Work out the finished part from the listing and answer in its coordinate system (mm). A direction names the side the tool comes from. Round coordinates to 2 decimals unless told otherwise and drop trailing zeros. Write each loop counter-clockwise with the first axis right and the second up, starting at its lowest first coordinate (ties: lowest second). Pieces come first, ordered by that corner, then holes.
1. A tool of negligible diameter and unlimited length cuts with its end or side. For faces 4 (the face through (20.35, 1.77, -24.81)), 5 (the face through (-22.72, 4.31, 20.69)), from which of +Z, -Z, +X, -X, +Y, -Y can it reach the whole face along a straight path? Write none if from no direction.
2. Find section D-D (y = 2.8). Write down the section's boundary in (x, z).
3. Find section C-C (x = -21.5). Write down the section's boundary in (y, z), and give its area (3 significant figures).
4. Find section B-B (x = 35). Write down the section's boundary in (y, z), and give its area (3 significant figures).
5. Straight lines are drawn through the part: probe 1 along X at (y, z) = (0.6, -22); probe 2 along X at (y, z) = (1.35, 23); probe 3 along Z at (x, y) = (24, 0.3). For each, find the intervals that lie inside material, in ascending order.
6. Find section A-A (z = -29). Write down the section's boundary in (x, y), and give its area (3 significant figures).
7. Flat-ended cylindrical pins translate along their axes: pin 1 Ø5.5 at (x, z) = (21.5, -22.04) entering from -Y; pin 2 Ø5 at (x, z) = (-35, -29) entering from +Y; pin 3 Ø2 at (x, y) = (-23, 4) entering from -Z. Find the tip coordinate at first contact, or state that the pin passes through.
8. Determine the mould class of faces 1 (the face through (-1, 1, -35)), 2 (the face through (-42.5, 1, 0)), 3 (the face through (34.1, 2.5, -18.7)) for opening direction X: pulls with the +X half, pulls with the -X half, needs draft (parallel to the pull), parting line crosses it, or undercut.
```python
from build123d import *

# Parameters (mm, degrees)
SKETCH1_W           = 85
SKETCH1_H           = 70
SKETCH1_R           = 1.5
BOSS_EXTRUDE1_DEPTH = 5
CUT_EXTRUDE1_REACH  = 57.283
SKETCH3_R           = 1.25
SKETCH4_R           = 3
CUT_EXTRUDE2_DEPTH  = 3.6
FILLET2_R           = 3


with BuildPart() as part:
    # Sketch1 → Boss-Extrude1 (new body)
    with BuildSketch(Plane(origin=(0, 0, 0), x_dir=(1, 0, 0), z_dir=(0, 1, 0))):
        Rectangle(SKETCH1_W, SKETCH1_H)
        with Locations(Location((-35, 29, 0), (0, 0, 270))):
            Circle(SKETCH1_R, mode=Mode.SUBTRACT)
        with Locations(Location((-37, -29, 0), (0, 0, 270))):
            Circle(SKETCH1_R, mode=Mode.SUBTRACT)
        with Locations(Location((35, 17.5, 0), (0, 0, 270))):
            Circle(SKETCH1_R, mode=Mode.SUBTRACT)
    extrude(amount=BOSS_EXTRUDE1_DEPTH)

    # Sketch3 → Cut-Extrude1 (cut, up to next)
    with BuildSketch(Plane(origin=(0, 5, 0), x_dir=(1, 0, 0), z_dir=(0, 1, 0)), mode=Mode.PRIVATE) as cut_extrude1_sk1:
        with Locations(Location((-21.5, 22.037196785, 0), (0, 0, 270))):
            Circle(SKETCH3_R)
    cut_extrude1_tool1 = extrude(cut_extrude1_sk1.sketch, amount=-CUT_EXTRUDE1_REACH, mode=Mode.PRIVATE) & part.part
    # Sketch3 → Cut-Extrude1 (cut, up to next)
    with BuildSketch(Plane(origin=(0, 5, 0), x_dir=(1, 0, 0), z_dir=(0, 1, 0)), mode=Mode.PRIVATE) as cut_extrude1_sk2:
        with Locations(Location((21.5, 22.037196785, 0), (0, 0, 270))):
            Circle(SKETCH3_R)
    cut_extrude1_tool2 = extrude(cut_extrude1_sk2.sketch, amount=-CUT_EXTRUDE1_REACH, mode=Mode.PRIVATE) & part.part
    # Sketch3 → Cut-Extrude1 (cut, up to next)
    with BuildSketch(Plane(origin=(0, 5, 0), x_dir=(1, 0, 0), z_dir=(0, 1, 0)), mode=Mode.PRIVATE) as cut_extrude1_sk3:
        with Locations(Location((-21.5, -20.962803215, 0), (0, 0, 270))):
            Circle(SKETCH3_R)
    cut_extrude1_tool3 = extrude(cut_extrude1_sk3.sketch, amount=-CUT_EXTRUDE1_REACH, mode=Mode.PRIVATE) & part.part
    # Sketch3 → Cut-Extrude1 (cut, up to next)
    with BuildSketch(Plane(origin=(0, 5, 0), x_dir=(1, 0, 0), z_dir=(0, 1, 0)), mode=Mode.PRIVATE) as cut_extrude1_sk4:
        with Locations(Location((21.5, -20.962803215, 0), (0, 0, 270))):
            Circle(SKETCH3_R)
    cut_extrude1_tool4 = extrude(cut_extrude1_sk4.sketch, amount=-CUT_EXTRUDE1_REACH, mode=Mode.PRIVATE) & part.part
    add(cut_extrude1_tool1.solids().sort_by_distance((-21.5, 5, -22.037197))[0], mode=Mode.SUBTRACT)
    add(cut_extrude1_tool2.solids().sort_by_distance((21.5, 5, -22.037197))[0], mode=Mode.SUBTRACT)
    add(cut_extrude1_tool3.solids().sort_by_distance((-21.5, 5, 20.962803))[0], mode=Mode.SUBTRACT)
    add(cut_extrude1_tool4.solids().sort_by_distance((21.5, 5, 20.962803))[0], mode=Mode.SUBTRACT)

    # Sketch4 → Cut-Extrude2 (cut)
    with BuildSketch(Plane.XZ):
        with Locations(Location((-21.5, 20.962803215, 0), (0, 0, 270))):
            Circle(SKETCH4_R)
        with Locations(Location((21.5, 20.962803215, 0), (0, 0, 270))):
            Circle(SKETCH4_R)
        with Locations(Location((21.5, -22.037196785, 0), (0, 0, 270))):
            Circle(SKETCH4_R)
        with Locations(Location((-21.5, -22.037196785, 0), (0, 0, 270))):
            Circle(SKETCH4_R)
    extrude(amount=-CUT_EXTRUDE2_DEPTH, mode=Mode.SUBTRACT)

    # Fillet2
    fillet2_edges = [part.edges().sort_by_distance(p)[0] for p in [
        (42.5, 5, 0),
        (0, 5, -35),
        (-42.5, 5, 0),
        (0, 5, 35),
    ]]
    fillet(fillet2_edges, radius=FILLET2_R)


solid = part.part
```
Worked answers:
1. face 4: -Y
1. face 5: +Y, -Y
2. outline: (-42.39, -34.89) - (42.39, -34.89) - (42.39, 34.89) - (-42.39, 34.89) - close; hole circle Ø3 at (-37, 29); hole circle Ø3 at (-35, -29); hole circle Ø6 at (-21.5, -22.04); hole circle Ø6 at (-21.5, 20.96); hole circle Ø6 at (21.5, -22.04); hole circle Ø6 at (21.5, 20.96); hole circle Ø3 at (35, -17.5)
3. outline: (0, -35) - (2, -35) arc R3 ccw to (5, -32) - (5, -23.29) - (3.6, -23.29) - (3.6, -25.04) - (0, -25.04) - close; (0, -19.04) - (3.6, -19.04) - (3.6, -20.79) - (5, -20.79) - (5, 19.71) - (3.6, 19.71) - (3.6, 17.96) - (0, 17.96) - close; (0, 23.96) - (3.6, 23.96) - (3.6, 22.21) - (5, 22.21) - (5, 32) arc R3 ccw to (2, 35) - (0, 35) - close
3. area: 296 mm2
4. outline: (0, -35) - (2, -35) arc R3 ccw to (5, -32) - (5, -19) - (0, -19) - close; (0, -16) - (5, -16) - (5, 32) arc R3 ccw to (2, 35) - (0, 35) - close
4. area: 331 mm2
5. probe 1: x = -42.5 to -24.5, -18.5 to 18.5, 24.5 to 42.5
5. probe 2: x = -42.5 to -23.7, -19.3 to 19.3, 23.7 to 42.5
5. probe 3: z = -35 to -23.7, -20.38 to 19.3, 22.62 to 35
6. outline: (-42.5, 0) - (-36.5, 0) - (-36.5, 5) - (-39.5, 5) arc R3 ccw to (-42.5, 2) - close; (-33.5, 0) - (42.5, 0) - (42.5, 2) arc R3 ccw to (39.5, 5) - (-33.5, 5) - close
6. area: 406 mm2
7. pin 1: stops at y = 3.6
7. pin 2: stops at y = 5
7. pin 3: stops at z = -34.83
8. face 1: needs draft
8. face 2: pulls with the -X half
8. face 3: undercut
